Answer from the drawing. Dimensions are ordinates in mm from the lowest x, y and z of the part. A direction names the side the tool comes from. Coordinates: 2 decimals unless noted, no trailing zeros. Order: outer loops, then holes, each group sorted by start corner. A loop starts at its lowest first (then second) coordinate and runs counter-clockwise, first axis right, second up. Notation, with made-up numbers: (87, -12.75) -> (108, -12.75) arc R36 ccw to (108, 22.25) -> close; hole circle Ø7 at (23.5, -23.5). An arc over 180 degrees is marked (long way). Answer as a JSON object with one key per item and string values. Group by question number.
1) A tool of negligible diameter and unlimited length cuts with its end or side. For the marked faces 1 and 2, from which of +Z, -Z, +X, -X, +Y, -Y can it reach the whole face along a straight path? Write none if from no direction.
2) Section C-C on y = 108 is taken. Determine the outline of the cut face in (x, z).
3) Section B-B on x = 59.5 is taken. Determine the outline of the cut face in (y, z).
4) Consider L1, parallel to Y at x = 86.5, z = 6 (1 decimal); L2, parallel to X at y = 103, z = 7; L3, parallel to Y at x = 160.5, z = 9.25. Determine where each line is inside the solid, lowest interval first.
5) Determine the mould class of the marked faces 3, 4, 5 and 6 for opening direction X: released by +X, released by -X, zero draft, split by the parting line, or undercut.
6) Section D-D on x = 152 is taken. Determine the outline of the cut face in (y, z).
7) Given pin 1 (1 mm diameter, centred on y = 92, z = 7.5, fed in from -X); pin 2 (1.5 mm diameter, centred on x = 140.5, z = 2.5, fed in from +Y) (1 decimal); pin 3 (3 mm diameter, centred on x = 116, z = 5.5, fed in from -Y), each flat-ended and moving along its own axis, determine where each tip first touches the part or whether it passes through.
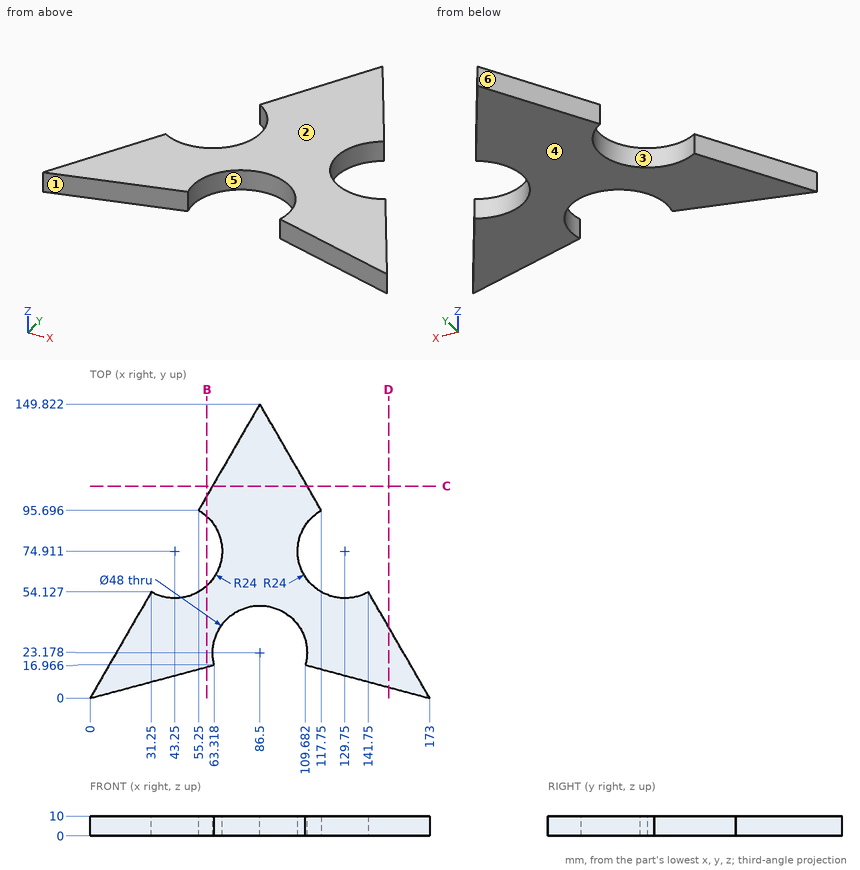
Worked answers:
{
 "1": {"face 1": "+Z, -Z, -Y", "face 2": "+Z, +X, -X, +Y, -Y"},
 "2": {"outline": "(62.35, 0) -> (110.65, 0) -> (110.65, 10) -> (62.35, 10) -> close"},
 "3": {"outline": "(15.94, 0) -> (57.25, 0) -> (57.25, 10) -> (15.94, 10) -> close; (92.57, 0) -> (103.06, 0) -> (103.06, 10) -> (92.57, 10) -> close"},
 "4": {"L1": "y = 47.2 to 149.8", "L2": "x = 59.47 to 113.53", "L3": "y = 3.35 to 21.65"},
 "5": {"face 3": "undercut", "face 4": "zero draft", "face 5": "undercut", "face 6": "released by -X"},
 "6": {"outline": "(5.63, 0) -> (36.37, 0) -> (36.37, 10) -> (5.63, 10) -> close"},
 "7": {"pin 1": "stops at x = 59.58", "pin 2": "stops at y = 53.8", "pin 3": "stops at y = 14.87"}
}
